```python
from build123d import *

# Parameters (mm, degrees)
F0_R     = 17.5
F1_DEPTH = 20
F2_R     = 10.927748
F3_DEPTH = 3
F5_DEPTH = 10
F6_W     = 0.44194
F6_H     = 0.254811


with BuildPart() as f1:
    # F0 (on Front) → F1 (new body)
    with BuildSketch(Plane.XZ):
        Circle(F0_R)
    extrude(amount=-F1_DEPTH)

    # F2 (on Front) → F3 (cut)
    with BuildSketch(Plane.XZ):
        with Locations((-16.442308, 13.46154)):
            Circle(F2_R)
    extrude(amount=-F3_DEPTH, mode=Mode.SUBTRACT)

    # F4 (on face) → F5 (cut)
    with BuildSketch(Plane(origin=(0, 20, 0), x_dir=(-1, 0, 0), z_dir=(0, 1, 0))):
        with BuildLine():
            ThreePointArc((-0.071881, 1.998708), (-1.388567, -1.439403), (2, 0))
            ThreePointArc((2, 0), (1.957133, 0.411864), (1.830368, 0.806073))
            Line((1.830368, 0.806073), (-0.071881, 1.998708))
        make_face()
    extrude(amount=-F5_DEPTH, mode=Mode.SUBTRACT)

    # F6 (on Right) → F7 (revolve, cut)
    with BuildSketch(Plane.YZ):
        with Locations((0.954671, 17.401108)):
            Rectangle(F6_W, F6_H)
    revolve(axis=Axis((0, 0, 0), (0, -1, 0)), mode=Mode.SUBTRACT)


solid = f1.part
```
Source: CAD feature listing. Evaluate the final solid. Frame: model axes, mm. A direction names the side the tool comes from. Coordinates: 2 decimals unless noted, no trailing zeros. Loops run counter-clockwise (first coordinate to the right, second up) from the corner with the lowest first, then second, coordinate; pieces in that order, holes last. Notation, with made-up numbers: M 9,69.5 L 44,69.5 A25 ccw 44,100.5 Z; hole C -30.5,-37.75 d3. An arc over 180 degrees is marked long. Put each result on its own line as item: value. Start each with the question number.
1) Ray query, L1, parallel to X at y = 14, z = 0; L2, parallel to Y at x = -9, z = 10.5; L3, parallel to Z at x = 0, y = 13. Return the intervals inside material, ascending. Write a range as from..to.
2) Contact query for flat-ended pins moving along their axis: pin 1 Ø5 at (x, z) = (10, -7.5) entering from -Y; pin 2 Ø3 at (x, z) = (0, 0) entering from +Y; pin 3 Ø5 at (x, y) = (5.5, 11) entering from -Z; pin 4 Ø1 at (x, y) = (12.5, 3) entering from +Z. Output: stop coordinate, or through.
3) Cut plane D-D on y = 4.5. Return the cut outline in (x, z).
4) Reachability of faces 4 (the face through (8.075, 10.456, -15.526)), 5 (the face through (-1.958, 15.07, 0.406)) from +Z, -Z, +X, -X, +Y, -Y: full face, straight path, thin tool, end or side. Return the list, or none.
5) Cut plane B-B on z = -10.5. Return the cut outline in (x, y).
6) Cut plane A-A on x = 11. Return the cut outline in (y, z), then the cut area to 3 significant figures.
7) Pull-direction query (Y, two-part tool) for faces 1 (the face through (0, 0, 0)), 2 (the face through (1.435, 15.07, -1.393)), 3 (the face through (12.96, 0.96, -11.42)); classes: pulls with the +Y half, pulls with the -Y half, needs draft (parallel to the pull), parting line crosses it, or undercut.
8) Cut plane C-C on y = 15.5. Return the cut outline in (x, z).
The answers:
1. L1: x = -17.5..-2, 2..17.5
1. L2: y = 3..20
1. L3: z = -17.5..-2, 1.95..17.5
2. pin 1: stops at y = 0
2. pin 2: stops at y = 10
2. pin 3: stops at z = -17.24
2. pin 4: stops at z = 12.74
3. outline: C 0,0 d35
4. face 4: +Y, -Y
4. face 5: +Y
5. outline: M -14,0 L 14,0 L 14,0.73 L 13.72,0.73 L 13.72,1.18 L 14,1.18 L 14,20 L -14,20 L -14,1.18 L -13.72,1.18 L -13.72,0.73 L -14,0.73 Z
6. outline: M 0,-13.61 L 0.73,-13.61 L 0.73,-13.32 L 1.18,-13.32 L 1.18,-13.61 L 20,-13.61 L 20,13.61 L 1.18,13.61 L 1.18,13.32 L 0.73,13.32 L 0.73,13.61 L 0,13.61 Z
6. area: 544 mm²
7. face 1: pulls with the -Y half
7. face 2: needs draft
7. face 3: undercut
8. outline: C 0,0 d35; hole M -2,0 A2 ccw long 0.07,2 L -1.83,0.81 A2 ccw Z
